from build123d import *

# Parameters (mm, degrees)
SKETCH_1_W          = 7.65
SKETCH_1_H          = 11
EXTRUDE_1_DEPTH     = 13.25
SKETCH_2_W          = 3.35
SKETCH_2_H          = 2
EXTRUDE_2_DEPTH     = 1.1
SKETCH_3_R          = 2.8
CUT_EXTRUDE_1_DEPTH = 3


with BuildPart() as part:
    # Эскиз1 → Бобышка-Вытянуть1 (new body)
    with BuildSketch(Plane.XY):
        Rectangle(SKETCH_1_W, SKETCH_1_H)
    extrude(amount=EXTRUDE_1_DEPTH)

    # Эскиз2 → Бобышка-Вытянуть2 (add)
    with BuildSketch(Plane(origin=(0, 5.5, 0), x_dir=(1, 0, 0), z_dir=(0, 1, 0))):
        with Locations((2.15, -4.85)):
            Rectangle(SKETCH_2_W, SKETCH_2_H)
    extrude_2 = extrude(amount=EXTRUDE_2_DEPTH)

    # Зеркальное отражение1: Бобышка-Вытянуть2 across plane
    add(extrude_2.mirror(Plane.ZX))

    # Эскиз3 → Вырез-Вытянуть1 (cut)
    with BuildSketch(Plane.XY.offset(13.25)):
        with Locations((0, 0.3)):
            Circle(SKETCH_3_R)
    extrude(amount=-CUT_EXTRUDE_1_DEPTH, mode=Mode.SUBTRACT)


solid = part.part
The model under review builds one solid part; all positions refer to its coordinate system, in mm. A direction names the side the tool comes from. Round coordinates to 2 decimals unless told otherwise and drop trailing zeros. Write each loop counter-clockwise with the first axis right and the second up, starting at its lowest first coordinate (ties: lowest second). Pieces come first, ordered by that corner, then holes. Notation, with made-up numbers: M 75,68.5 L 117,68.5 A31 cw 117,104.5 Z; hole C 61,20.25 d2. An arc over 180 degrees is marked long. Answer as CSV lines item,"result". Start each with the question number.
Q1. Consider section A-A, the plane z = 11.5. Give the boundary of the cut face in (x, y) (3 decimals), then the cut area to 3 significant figures.
Q2. Consider section B-B, the plane y = 0.3. Give the boundary of the cut face in (x, z) (3 decimals), then the cut area to 3 significant figures.
Q3. Wall thickness on line 1 along Y through (x, z) = (0, 10.95); line 2 along Y through (x, z) = (-1.5, 4.75); line 3 along Z through (x, y) = (0.75, 0.5): over which ranges is each line inside the solid? List them lowest first.
Q4. Consider section D-D, the plane x = 2. Give the boundary of the cut face in (y, z), then the cut area to 3 significant figures.
Q5. Tool access review of faces 1 (the face through (0, 0, 10.25)), 2 (the face through (0.475, -6, 5)), 3 (the face through (0.475, 6, 5)), 4 (the face through (2, 6, 3.85)), 5 (the face through (2, 6, 5.85)): name each direction out of +Z, -Z, +X, -X, +Y, -Y from which nothing blocks a thin tool from reaching the whole face with its end or side.
Q6. Consider section C-C, the plane z = 4.25. Give the boundary of the cut face in (x, y) (3 decimals).
Q7. The part is to be moulded in two halves that separate along X. For faces 6 (the face through (3.825, 0, 7)), 7 (the face through (2, -6, 5.85)), 8 (the face through (-3.825, 0, 7)), 9 (the face through (1.51, 2.66, 11.77)), say which applies: +X half, -X half, draft (parallel to the pull), parting line (faces both ways), or undercut.
Q8. Clearance check with flat-ended pins moving along their axes: P1, Ø0.9, axis at x = 2.5, y = 6, coming from the +Z side; P2, Ø0.9, axis at x = 3, y = -6, coming from the -Z side; P3, Ø4, axis at x = 2.5, z = 9, coming from the -Y side. State where each tip first meets the part, or that it passes through.
Result set:
1,outline,"M -3.825,-5.5 L 3.825,-5.5 L 3.825,5.5 L -3.825,5.5 Z; hole C 0,0.3 d5.6"
1,area,"59.5 mm²"
2,outline,"M -3.825,0 L 3.825,0 L 3.825,13.25 L 2.8,13.25 L 2.8,10.25 L -2.8,10.25 L -2.8,13.25 L -3.825,13.25 Z"
2,area,"84.6 mm²"
3,line 1,"y = -5.5 to -2.5, 3.1 to 5.5"
3,line 2,"y = -5.5 to 5.5"
3,line 3,"z = 0 to 10.25"
4,outline,"M -6.6,3.85 L -5.5,3.85 L -5.5,0 L 5.5,0 L 5.5,3.85 L 6.6,3.85 L 6.6,5.85 L 5.5,5.85 L 5.5,13.25 L 2.26,13.25 L 2.26,10.25 L -1.66,10.25 L -1.66,13.25 L -5.5,13.25 L -5.5,5.85 L -6.6,5.85 Z"
4,area,"138 mm²"
5,face 1,"+Z"
5,face 2,"+Z, -Z, -X, -Y"
5,face 3,"+Z, -Z, -X, +Y"
5,face 4,"-Z, +X, -X, +Y"
5,face 5,"+Z, +X, -X, +Y"
6,outline,"M -3.825,-5.5 L 0.475,-5.5 L 0.475,-6.6 L 3.825,-6.6 L 3.825,6.6 L 0.475,6.6 L 0.475,5.5 L -3.825,5.5 Z"
7,face 6,"+X half"
7,face 7,"draft"
7,face 8,"-X half"
7,face 9,"undercut"
8,P1,"stops at z = 5.85"
8,P2,"stops at z = 3.85"
8,P3,"stops at y = -5.5"
